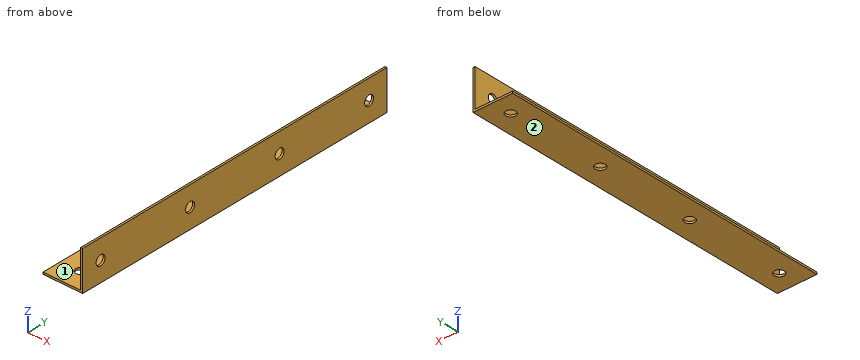
from build123d import *

# Parameters (mm, degrees)
F1_DEPTH = 215.9
F2_R     = 3.175
F3_DEPTH = 25.401
F4_R     = 3.175
F5_DEPTH = 25.4


with BuildPart() as f1:
    # F0 (on Front) → F1 (new body)
    with BuildSketch(Plane.XZ):
        Polygon((-12.7, -11.43), (-12.7, -12.7), (12.7, -12.7), (12.7, 12.7), (11.43, 12.7), (11.43, -11.43), align=None)
    extrude(amount=F1_DEPTH)

    # F2 (on face) → F3 (cut, through all)
    with BuildSketch(Plane(origin=(0, 0, -12.7), x_dir=(1, 0, 0), z_dir=(0, 0, -1))):
        with Locations((0, 203.2)):
            Circle(F2_R)
        with Locations((0, 139.7)):
            Circle(F2_R)
        with Locations((0, 76.2)):
            Circle(F2_R)
        with Locations((0, 12.7)):
            Circle(F2_R)
    extrude(amount=-F3_DEPTH, mode=Mode.SUBTRACT)

    # F4 (on face) → F5 (cut)
    with BuildSketch(Plane.YZ.offset(12.7)):
        with Locations((-139.7, 0)):
            Circle(F4_R)
        with Locations((-203.2, 0)):
            Circle(F4_R)
        with Locations((-76.2, 0)):
            Circle(F4_R)
        with Locations((-12.7, 0)):
            Circle(F4_R)
    extrude(amount=-F5_DEPTH, mode=Mode.SUBTRACT)


solid = f1.part
Work out the finished part from the listing and answer in its coordinate system (mm). Face numbers are marked on the shaded views. A direction names the side the tool comes from. Round coordinates to 2 decimals unless told otherwise and drop trailing zeros. Order: outer loops, then holes, each group sorted by start corner. A loop starts at its lowest first (then second) coordinate and runs counter-clockwise, first axis right, second up. Notation, with made-up numbers: M 59.5,-19 L 69.5,-19 A12 cw 69.5,-9 Z; hole C 56,20.5 d1. An arc over 180 degrees is marked long. Put each result on its own line as item: value. Start each with the question number.
Q1. Straight lines are drawn through the part: L1, parallel to Y at x = 0, z = -11.95 (3 decimals); L2, parallel to Z at x = -9.25, y = -19; L3, parallel to X at y = -12.7, z = -12.4 (3 decimals). For each, find the intervals that lie inside material, in ascending order. Write a range as [from, to].
Q2. Flat-ended cylindrical pins translate along their axes: pin 1 (12 mm diameter, centred on y = -114, z = -1.5, fed in from -X); pin 2 (8 mm diameter, centred on x = 6.5, y = -25.5, fed in from +Z). Find the tip coordinate at first contact, or state that the pin passes through.
Q3. Section B-B, the plane y = -12.7 is taken. Write down the section's boundary in (x, z) (3 decimals).
Q4. Section D-D, the plane y = -192.5 is taken. Write down the section's boundary in (x, z), and give its area (3 significant figures).
Q5. Section A-A, the plane x = 0 is taken. Write down the section's boundary in (y, z) (3 decimals).
Q6. A tool of negligible diameter and unlimited length cuts with its end or side. For the marked faces 1 and 2, from which of +Z, -Z, +X, -X, +Y, -Y can it reach the whole face along a straight path? Write none if from no direction.
Q7. Section C-C, the plane z = 0 is taken. Write down the section's boundary in (x, y) (3 decimals), and give its area (3 significant figures).
Findings below:
1. L1: y = [-215.9, -206.375], [-200.025, -142.875], [-136.525, -79.375], [-73.025, -15.875], [-9.525, 0]
1. L2: z = [-12.7, -11.43]
1. L3: x = [-12.7, -3.175], [3.175, 12.7]
2. pin 1: stops at x = 11.43
2. pin 2: stops at z = -11.43
3. outline: M -12.7,-12.7 L -3.175,-12.7 L -3.175,-11.43 L -12.7,-11.43 Z; M 3.175,-12.7 L 12.7,-12.7 L 12.7,-3.175 L 11.43,-3.175 L 11.43,-11.43 L 3.175,-11.43 Z; M 11.43,3.175 L 12.7,3.175 L 12.7,12.7 L 11.43,12.7 Z
4. outline: M -12.7,-12.7 L 12.7,-12.7 L 12.7,12.7 L 11.43,12.7 L 11.43,-11.43 L -12.7,-11.43 Z
4. area: 62.9 mm^2
5. outline: M -215.9,-12.7 L -206.375,-12.7 L -206.375,-11.43 L -215.9,-11.43 Z; M -200.025,-12.7 L -142.875,-12.7 L -142.875,-11.43 L -200.025,-11.43 Z; M -136.525,-12.7 L -79.375,-12.7 L -79.375,-11.43 L -136.525,-11.43 Z; M -73.025,-12.7 L -15.875,-12.7 L -15.875,-11.43 L -73.025,-11.43 Z; M -9.525,-12.7 L 0,-12.7 L 0,-11.43 L -9.525,-11.43 Z
6. face 1: +Z, -X, +Y, -Y
6. face 2: -Z, +X, -X, +Y, -Y
7. outline: M 11.43,-215.9 L 12.7,-215.9 L 12.7,-206.375 L 11.43,-206.375 Z; M 11.43,-200.025 L 12.7,-200.025 L 12.7,-142.875 L 11.43,-142.875 Z; M 11.43,-136.525 L 12.7,-136.525 L 12.7,-79.375 L 11.43,-79.375 Z; M 11.43,-73.025 L 12.7,-73.025 L 12.7,-15.875 L 11.43,-15.875 Z; M 11.43,-9.525 L 12.7,-9.525 L 12.7,0 L 11.43,0 Z
7. area: 242 mm^2
